Design review of the part built by this model. Coordinates are the model's own, in mm. A direction names the side the tool comes from. Round coordinates to 2 decimals unless told otherwise and drop trailing zeros. Write each loop counter-clockwise with the first axis right and the second up, starting at its lowest first coordinate (ties: lowest second). Pieces come first, ordered by that corner, then holes. Notation, with made-up numbers: (-21, 76.25) -> (6, 76.25) arc R27 ccw to (6, 107.25) -> close; hole circle Ø6 at (53.5, 45.5). An arc over 180 degrees is marked (long way). Write item = value, one per line. Start each with the question number.
Item 1: Mouldability with a two-part tool opening along Y and no side actions: class faces 3 (the cylindrical face through (6.386, -7.199, -20.685)), 4 (the flat face through (2, -20, -30)), 5 (the cylindrical face through (0.9, -2.46, -0.86)), 6 (the flat face through (21, 0, -7)) as released by +Y, released by -Y, zero draft, split by the parting line, or undercut.
Item 2: To check wall thickness, follow L1, parallel to Y at x = 15.5, z = -11; L2, parallel to Z at x = 37, y = -3; L3, parallel to Z at x = 37, y = -1.8. State the ranges of each line that lie inside material, in increasing order.
Item 3: Add section B-B, the plane x = 13. State the section outline as (y, z) points.
Item 4: Add section A-A, the plane z = -5. State the section outline as (x, y) points.
Item 5: Add section D-D, the plane x = 22. State the section outline as (y, z) points, then the cut area to 3 significant figures.
Item 6: Machinability: for faces 1 (the cylindrical face through (6.43, -29.1, -42.59)), 2 (the flat face through (21, -5, -7)), which of the approach directions +Z, -Z, +X, -X, +Y, -Y give a long, thin tool a straight path to every point of the face, cutting with its end or side? Answer none if there is none.
Item 7: Add section C-C, the plane x = 37.5. State the section outline as (y, z) points, then the cut area to 3 significant figures.
Item 8: For pin 1 Ø1 at (x, z) = (29, -15) entering from -Y; pin 2 Ø2.5 at (x, z) = (37, -5) entering from -Y; pin 3 Ø6 at (x, y) = (33, -11) entering from -Z; pin 4 Ø12 at (x, z) = (12.5, -7.5) entering from -Y, all flat-tipped, find the tip position at first contact; note any pin that passes through.
from build123d import *

# Parameters (mm, degrees)
F0_R     = 1.5
F1_DEPTH = 5
F3_DEPTH = 42
F4_R     = 1.5
F4_R_2   = 18
F5_DEPTH = 5


with BuildPart() as f1:
    # F0 (on Front) → F1 (new body)
    with BuildSketch(Plane.XZ):
        with BuildLine():
            Line((39, 0), (3, 0))
            ThreePointArc((3, 0), (0.87868, -0.87868), (0, -3))
            Line((0, -3), (0, -15))
            Line((0, -15), (42, -15))
            Line((42, -15), (42, -3))
            ThreePointArc((42, -3), (41.12132, -0.87868), (39, 0))
        make_face()
        with Locations((5, -5)):
            Circle(F0_R, mode=Mode.SUBTRACT)
        with Locations((37, -5)):
            Circle(F0_R, mode=Mode.SUBTRACT)
    extrude(amount=F1_DEPTH)

    # F2 (on face) → F3 (join)
    with BuildSketch(Plane(origin=(0, 0, 0), x_dir=(0, -1, 0), z_dir=(-1, 0, 0))):
        Polygon((34.698485, -44.698485), (5, -15), (0, -15), (1.464466, -18.535534), (31.162951, -48.234019), align=None)
    extrude(amount=-F3_DEPTH)

    # F4 (on face) → F5 (cut)
    with BuildSketch(Plane(origin=(0, 5, -5), x_dir=(1, 0, 0), z_dir=(0, -0.707107, 0.707107))):
        with Locations((37, -19.142136)):
            Circle(F4_R)
        with Locations((37, -51.142136)):
            Circle(F4_R)
        with Locations((5, -51.142136)):
            Circle(F4_R)
        with Locations((5, -19.142136)):
            Circle(F4_R)
        with Locations((21, -35.142136)):
            Circle(F4_R_2)
    extrude(amount=-F5_DEPTH, mode=Mode.SUBTRACT)


solid = f1.part
Result set:
q1.face_3 = undercut
q1.face_4 = released by -Y
q1.face_5 = zero draft
q1.face_6 = released by +Y
q2.L1 = -5 to 0
q2.L2 = -20.07 to -6.5, -3.5 to 0
q2.L3 = -18.87 to -6.5, -3.5 to 0
q3.outline = (-34.7, -44.7) -> (-31.16, -48.23) -> (-27.72, -44.79) -> (-31.25, -41.25) -> close; (-8.45, -18.45) -> (-4.91, -21.98) -> (-1.46, -18.54) -> (0, -15) -> (0, 0) -> (-5, 0) -> (-5, -15) -> close
q4.outline = (0, -5) -> (3.5, -5) -> (3.5, 0) -> (0, 0) -> close; (6.5, -5) -> (35.5, -5) -> (35.5, 0) -> (6.5, 0) -> close; (38.5, -5) -> (42, -5) -> (42, 0) -> (38.5, 0) -> close
q5.outline = (-34.7, -44.7) -> (-31.16, -48.23) -> (-29.02, -46.09) -> (-32.56, -42.56) -> close; (-7.14, -17.14) -> (-3.61, -20.68) -> (-1.46, -18.54) -> (0, -15) -> (0, 0) -> (-5, 0) -> (-5, -15) -> close
q5.area = 114 mm²
q6.face_1 = none
q6.face_2 = +Z, +X, -X, -Y
q7.outline = (-34.7, -44.7) -> (-31.16, -48.23) -> (-28.63, -45.7) -> (-32.16, -42.16) -> close; (-30.16, -40.16) -> (-26.63, -43.7) -> (-21.4, -38.47) -> (-24.94, -34.94) -> close; (-14.76, -24.76) -> (-11.23, -28.3) -> (-6, -23.07) -> (-9.54, -19.54) -> close; (-7.54, -17.54) -> (-4, -21.07) -> (-1.46, -18.54) -> (0, -15) -> (0, -6.41) -> (-5, -6.41) -> (-5, -15) -> close; (-5, -3.59) -> (0, -3.59) -> (0, 0) -> (-5, 0) -> close
q7.area = 179 mm²
q8.pin_1 = -5.5
q8.pin_2 = through
q8.pin_3 = -25.32
q8.pin_4 = -5
